Autodesk Inventor part; units mm, degrees
ref_plane "YZ Plane" through (0, 0, 0) normal (1, 0, 0) x (0, 1, 0)
ref_plane "XZ Plane" through (0, 0, 0) normal (0, 1, 0) x (-1, 0, 0)
ref_plane "XY Plane" through (0, 0, 0) normal (0, 0, 1) x (1, 0, 0)
sketch "Sketch1" plane through (0, 0, 0) normal (0, 0, 1) x (1, 0, 0)
  line L0 (-54, -37.5) -> (54, -37.5)
  line L1 (54, -37.5) -> (54, 37.5)
  line L2 (54, 37.5) -> (-54, 37.5)
  line L3 (-54, 37.5) -> (-54, -37.5)
  line L4 (-54, -37.5) -> (54, 37.5) construction
  line L5 (54, -37.5) -> (-54, 37.5) construction
  point P0 (0, 0)
  dimension "d0" = 108
  dimension "d1" = 75
extrude "Extrusion1" add sketch "Sketch1" along normal mid plane 6.35
sketch "Sketch3" plane through (0, 0, 3.175) normal (0, 0, 1) x (1, 0, 0)
  circle A0 centre (0, -5.5) radius 7
  line L0 (-54, -37.5) -> (54, -37.5) construction
  circle A1 centre (-10.6066, 5.1066) radius 2
  line L1 (0, -5.5) -> (-54, -5.5) construction
  line L2 (-54, -37.5) -> (-54, 37.5) construction
  line L3 (0, -5.5) -> (-10.6066, 5.1066) construction
  circle A2 centre (-10.6066, -16.1066) radius 2
  circle A3 centre (10.6066, -16.1066) radius 2
  circle A4 centre (10.6066, 5.1066) radius 2
  line L4 (0, -5.5) -> (-15.5563, 10.0563) construction
  circle A5 centre (-15.5563, 10.0563) radius 2
  circle A6 centre (-15.5563, -21.0563) radius 2
  circle A7 centre (15.5563, -21.0563) radius 2
  circle A8 centre (15.5563, 10.0563) radius 2
  circle A9 centre (-28.0623, -33.5623) radius 4.1
  point P0 (0, 0)
  point P1 (0, -37.5)
  dimension "d16" = 14
  dimension "d17" = 32
  dimension "d18" = 4
  dimension "d19" = 45
  dimension "d20" = 15
  dimension "d23" = 360
  dimension "d25" = 22
  dimension "d26" = 4
  dimension "d29" = 360
  dimension "d65" = 8.2
extrude "Extrusion3" cut sketch "Sketch3" against normal through all contours A0 | A1 | A2 | A3 | A4 | A5 | A6 | A7 | A8
sketch "Sketch5" plane through (0, 0, 3.175) normal (0, 0, 1) x (1, 0, 0)
  circle A0 centre (-48, -29.5) radius 3
  line L0 (-54, 37.5) -> (-54, -37.5) construction
  line L1 (-54, -37.5) -> (54, -37.5) construction
  circle A1 centre (-34, -29.5) radius 3
  circle A2 centre (-34, -13.5) radius 4
  circle A3 centre (-48, -13.5) radius 4
  circle A4 centre (-34, 0.5) radius 4
  circle A5 centre (-48, 0.5) radius 4
  line L2 (-54, 37.5) -> (54, 37.5)
  line L3 (0, 37.5) -> (0, -37.5) construction
  line L4 (54, -37.5) -> (-54, -37.5) construction
  circle A6 centre (48, -29.5) radius 3
  circle A7 centre (34, -29.5) radius 3
  circle A8 centre (34, -13.5) radius 4
  circle A9 centre (48, -13.5) radius 4
  circle A10 centre (34, 0.5) radius 4
  circle A11 centre (48, 0.5) radius 4
  point P0 (0, 0)
  dimension "d45" = 6
  dimension "d46" = 6
  dimension "d47" = 8
  dimension "d48" = 6
  dimension "d49" = 14
  dimension "d50" = 8
  dimension "d51" = 16
  dimension "d52" = 8
  dimension "d53" = 8
  dimension "d54" = 14
  dimension "d55" = 8
extrude "Extrusion5" cut sketch "Sketch5" against normal through all
properties part number "FirstStageMotorPlate"
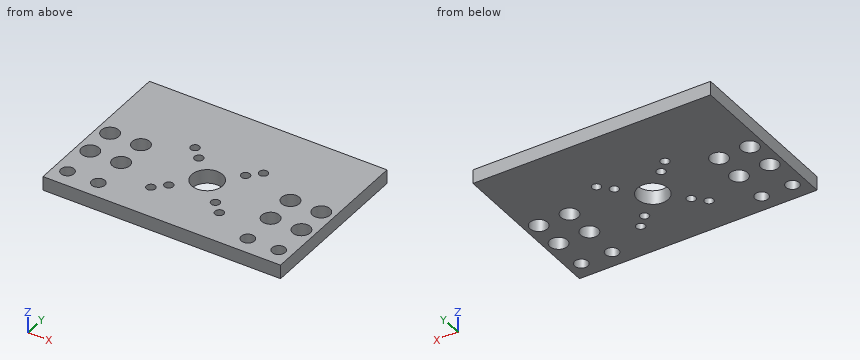
CAD build for the part. Positions are in the model's coordinates, mm. Coordinates: 2 decimals unless noted, no trailing zeros. Order: outer loops, then holes, each group sorted by start corner. A loop starts at its lowest first (then second) coordinate and runs counter-clockwise, first axis right, second up. Notation, with made-up numbers: (65, 11.5) -> (79, 11.5) arc R18 ccw to (79, 16.5) -> close; hole circle Ø8 at (81.25, 46.5). An arc over 180 degrees is marked (long way). Use one line per item in the form item = value. Start each with the question number.
1) Drop a flat-ended pin along its axis: pin 1 (7 mm diameter, centred on x = -48, y = -13.5, fed in from +Z). Give the stop position or say it passes through.
2) Band-saw the part on A-A on x = -34. Give the cut face in (y, z) (3 decimals), then the cut area to 3 significant figures.
3) Drill centre lines: L1, parallel to Y at x = -48, z = -1.5; L2, parallel to Y at x = 15.5, z = -0.5; L3, parallel to X at y = -21.5, z = -1.75. Where is each one in solid material? Low to high. Write a range as [from, to].
4) Band-saw the part on C-C on y = -29.5. Give the cut face in (x, z) (3 decimals).
5) Band-saw the part on B-B on y = -5.5. Give the cut face in (x, z) (3 decimals).
6) Band-saw the part on D-D on z = 0.5. State how many separate pieces and enclosed holes the cut face has, then the cut area to 3 significant figures.
Entries:
q1.pin_1 = through
q2.outline = (-37.5, -3.175) -> (-32.5, -3.175) -> (-32.5, 3.175) -> (-37.5, 3.175) -> close; (-26.5, -3.175) -> (-17.5, -3.175) -> (-17.5, 3.175) -> (-26.5, 3.175) -> close; (-9.5, -3.175) -> (-3.5, -3.175) -> (-3.5, 3.175) -> (-9.5, 3.175) -> close; (4.5, -3.175) -> (37.5, -3.175) -> (37.5, 3.175) -> (4.5, 3.175) -> close
q2.area = 337 mm2
q3.L1 = [-37.5, -32.5], [-26.5, -17.5], [-9.5, -3.5], [4.5, 37.5]
q3.L2 = [-37.5, -23.06], [-19.06, 8.06], [12.06, 37.5]
q3.L3 = [-54, -17.51], [-13.61, 13.61], [17.51, 54]
q4.outline = (-54, -3.175) -> (-51, -3.175) -> (-51, 3.175) -> (-54, 3.175) -> close; (-45, -3.175) -> (-37, -3.175) -> (-37, 3.175) -> (-45, 3.175) -> close; (-31, -3.175) -> (31, -3.175) -> (31, 3.175) -> (-31, 3.175) -> close; (37, -3.175) -> (45, -3.175) -> (45, 3.175) -> (37, 3.175) -> close; (51, -3.175) -> (54, -3.175) -> (54, 3.175) -> (51, 3.175) -> close
q5.outline = (-54, -3.175) -> (-7, -3.175) -> (-7, 3.175) -> (-54, 3.175) -> close; (7, -3.175) -> (54, -3.175) -> (54, 3.175) -> (7, 3.175) -> close
q6.separate_pieces = 1
q6.enclosed_holes = 21
q6.area = 7,330 mm2
